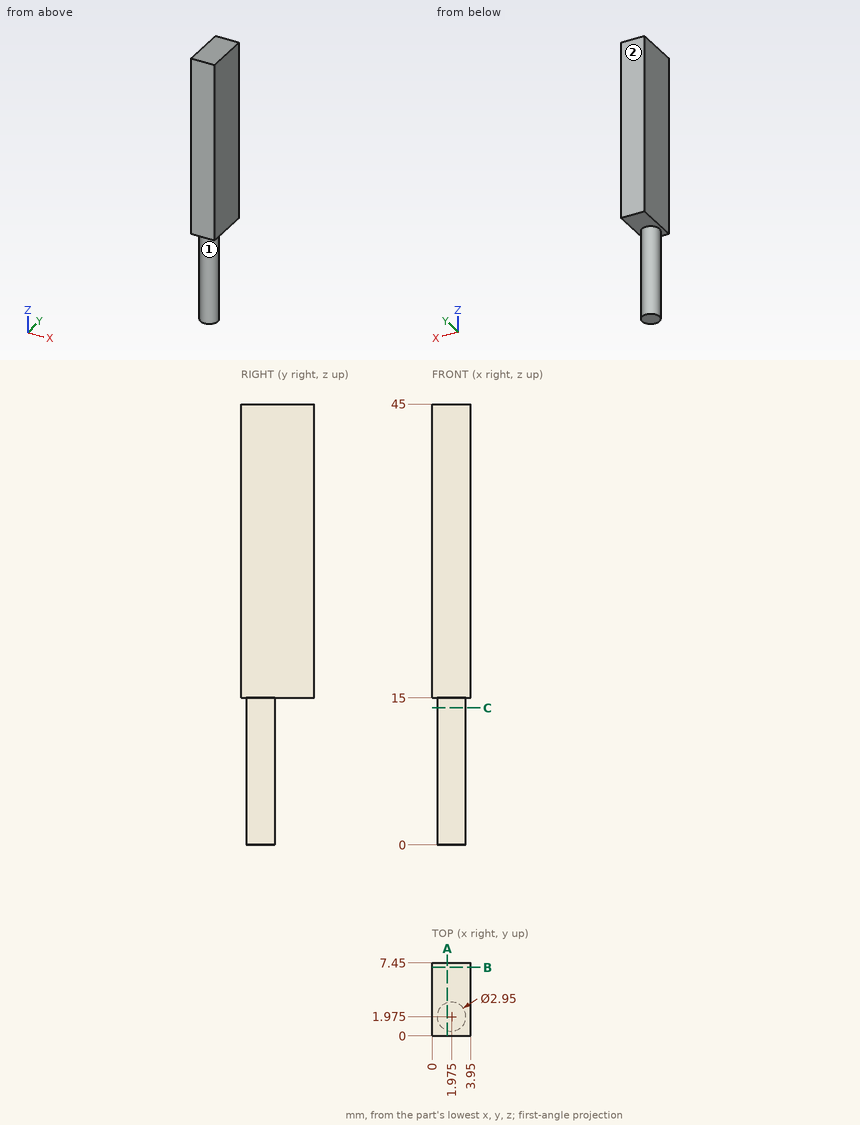
Input: dimensioned drawing with shaded views. Units: mm. Origin: part minimum x, y, z. A direction names the side the tool comes from. Give positions to 0.01 mm unless a question says otherwise; leave off trailing zeros. Write each loop counter-clockwise with the first axis right and the second up, starting at its lowest first coordinate (ties: lowest second). Pieces come first, ordered by that corner, then holes. Notation, with made-up numbers: (43, -17) -> (48, -17) arc R24 cw to (48, -5) -> close; hole circle Ø4 at (7.25, -10.5). An arc over 180 degrees is marked (long way). Return JSON: item names as keys, results as strings. Group by question number.
1. Section A-A, the plane x = 1.55. Output: boundary loops of the cut face in (y, z).
2. Section B-B, the plane y = 7. Output: boundary loops of the cut face in (x, z), then the cut area to 4 significant figures.
3. Access query for the marked faces 1 and 2. Directions: +Z, -Z, +X, -X, +Y, -Y. A direction counts if a zero-diameter tool reaches every point of the face in a straight line with its end or side. Return the directions, or none.
4. Pin query (flat end, axial travel): pin 1 Ø2 at (y, z) = (6, 27.5) entering from -X; pin 2 Ø1 at (x, z) = (2, 13.5) entering from -Y. Return the tip coordinate at first contact, or that it passes through.
5. Section C-C, the plane z = 14. Output: boundary loops of the cut face in (x, y) (3 decimals).
6. Material intervals for line 1 (Z direction, x = 2.35, y = 6); line 2 (Y direction, x = 2.3, z = 12); line 3 (Y direction, x = 2.5, z = 5), sorted ascending. Write a range as from..to.
Determined:
{
 "1": {"outline": "(0, 15) -> (0.56, 15) -> (0.56, 0) -> (3.39, 0) -> (3.39, 15) -> (7.45, 15) -> (7.45, 45) -> (0, 45) -> close"},
 "2": {"outline": "(0, 15) -> (3.95, 15) -> (3.95, 45) -> (0, 45) -> close", "area": "118.5 mm2"},
 "3": {"face 1": "-Z", "face 2": "+Z, -Z, +X, -X, +Y"},
 "4": {"pin 1": "stops at x = 0", "pin 2": "stops at y = 0.5"},
 "5": {"outline": "circle Ø2.95 at (1.975, 1.975)"},
 "6": {"line 1": "z = 15..45", "line 2": "y = 0.54..3.41", "line 3": "y = 0.6..3.35"}
}
